Check sheet for the modelled part. Datum: model origin and axes. Units: mm. Coordinates: 2 decimals unless noted, no trailing zeros. Write each loop counter-clockwise with the first axis right and the second up, starting at its lowest first coordinate (ties: lowest second). Pieces come first, ordered by that corner, then holes. Notation, with made-up numbers: (80.25, 8.5) - (96.25, 8.5) arc R20 cw to (96.25, 33.5) - close; hole circle Ø4 at (27, 40.25). An arc over 180 degrees is marked (long way). Write each question's results on one line, items separated by ' | '.
from build123d import *

# Parameters (mm, degrees)
F0_W     = 304.8
F0_H     = 254
F1_DEPTH = 6.35
F2_R     = 15.24
F3_DEPTH = 12.701
F4_R     = 3.175
F5_DEPTH = 12.701


with BuildPart() as f1:
    # F0 (on Top) → F1 (new body, symmetric)
    with BuildSketch(Plane.XY):
        Rectangle(F0_W, F0_H)
    extrude(amount=F1_DEPTH, both=True)

    # F2 (on face) → F3 (cut, through all)
    with BuildSketch(Plane.XY.offset(6.35)):
        Circle(F2_R)
    extrude(amount=-F3_DEPTH, mode=Mode.SUBTRACT)

    # F4 (on face) → F5 (cut, through all)
    with BuildSketch(Plane.XY.offset(6.35)):
        with Locations((-101.6, 0)):
            Circle(F4_R)
        with Locations((101.6, 0)):
            Circle(F4_R)
    extrude(amount=-F5_DEPTH, mode=Mode.SUBTRACT)


solid = f1.part
1. Go/stop test with a flat-tipped pin: pin 1 (10 mm diameter, centred on x = 101.6, y = 0, fed in from +Z). Record where the tip stops, or that it passes through.
Values follow:
pin 1: stops at z = 6.35
2. Draft check along Y on faces 1 (the flat face through (152.4, -2, 0)), 2 (the flat face through (-2, -127, 0)), 3 (the cylindrical face through (98.43, 0.14, 0.09)), 4 (the flat face through (-2, 127, 0)). Enter one of: pulls with the +Y half, pulls with the -Y half, needs draft (parallel to the pull), parting line crosses it, or undercut.
Values follow:
face 1: needs draft | face 2: pulls with the -Y half | face 3: undercut | face 4: pulls with the +Y half
3. Sectioned sample at A-A (x = 0). Record the cut outline in (y, z).
Values follow:
outline: (-127, -6.35) - (-15.24, -6.35) - (-15.24, 6.35) - (-127, 6.35) - close; (15.24, -6.35) - (127, -6.35) - (127, 6.35) - (15.24, 6.35) - close
4. Material ranges on L1, parallel to Y at x = 101.6, z = 2.75 (3 decimals); L2, parallel to Y at x = 0, z = 1.25, recorded low to high. Write a range as [from, to].
Values follow:
L1: y = [-127, -3.175], [3.175, 127] | L2: y = [-127, -15.24], [15.24, 127]
